Part model, mm, in its own coordinate system. Face numbers are marked on the shaded views. A direction names the side the tool comes from. Round coordinates to 2 decimals unless told otherwise and drop trailing zeros. Loops run counter-clockwise (first coordinate to the right, second up) from the corner with the lowest first, then second, coordinate; pieces in that order, holes last. Notation, with made-up numbers: (88.5, 33.5) - (132.5, 33.5) arc R9 ccw to (132.5, 40.5) - close; hole circle Ø5 at (31.5, 37). An arc over 180 degrees is marked (long way). Put each result on its own line as item: value.
from build123d import *

# Parameters (mm, degrees)
SKETCH1_W                  = 76.2
SKETCH1_H                  = 63.5
BOSS_EXTRUDE1_DEPTH        = 14.2875
SKETCH2_W                  = 50.8
SKETCH2_H                  = 36.1
CUT_EXTRUDE1_DEPTH         = 19.05
M10X1_5_TAPPED_HOLE1_D     = 8.5
M10X1_5_TAPPED_HOLE1_DEPTH = 22.446342369
M10X1_5_TAPPED_HOLE1_TIP   = 2.553657631
SKETCH16_W                 = 3.724215622
SKETCH16_H                 = 1.92405
FILLET2_R                  = 3.175
F_4_40_TAPPED_HOLE2_D      = 2.2606
F_4_40_TAPPED_HOLE2_DEPTH  = 6.920847242
F_4_40_TAPPED_HOLE2_TIP    = 0.679152758
FILLET3_R                  = 4
F_4_40_TAPPED_HOLE3_D      = 2.2606
F_4_40_TAPPED_HOLE3_DEPTH  = 4.320847242
F_4_40_TAPPED_HOLE3_TIP    = 0.679152758
F_8_32_TAPPED_HOLE1_D      = 3.4544
F_8_32_TAPPED_HOLE1_DEPTH  = 9.672193539
F_8_32_TAPPED_HOLE1_TIP    = 1.037806461


with BuildPart() as part:
    # Sketch1 → Boss-Extrude1 (new body, symmetric)
    with BuildSketch(Plane(origin=(0, 0, 0), x_dir=(1, 0, 0), z_dir=(0, 1, 0))):
        Rectangle(SKETCH1_W, SKETCH1_H)
    extrude(amount=BOSS_EXTRUDE1_DEPTH, both=True)

    # Sketch2 → Cut-Extrude1 (cut)
    with BuildSketch(Plane(origin=(0, 14.2875, 0), x_dir=(1, 0, 0), z_dir=(0, 1, 0))):
        Rectangle(SKETCH2_W, SKETCH2_H)
    extrude(amount=-CUT_EXTRUDE1_DEPTH, mode=Mode.SUBTRACT)

    # M10x1.5 Tapped Hole1
    with Locations(Plane(origin=(-21.9, 4.2875, -31.75), x_dir=(-1, 0, 0), z_dir=(0, 0, -1))):
        with Locations((0, 0)):
            Hole(M10X1_5_TAPPED_HOLE1_D / 2, depth=M10X1_5_TAPPED_HOLE1_DEPTH)
            with Locations((0, 0, -(M10X1_5_TAPPED_HOLE1_DEPTH + M10X1_5_TAPPED_HOLE1_TIP / 2))):  # 118° drill point
                Cone(0, M10X1_5_TAPPED_HOLE1_D / 2, M10X1_5_TAPPED_HOLE1_TIP, mode=Mode.SUBTRACT)

    # Cut-Sweep1: sweep along a path in Sketch14
    with BuildLine(Plane(origin=(0, 14.2875, 0), x_dir=(1, 0, 0), z_dir=(0, 1, 0))) as cut_sweep1_path:
        Line((-21.4, 20.05), (21.4, 20.05))
        ThreePointArc((21.4, 20.05), (25.642640687, 18.292640687), (27.4, 14.05))
        Line((27.4, 14.05), (27.4, -14.05))
        ThreePointArc((27.4, -14.05), (25.642640687, -18.292640687), (21.4, -20.05))
        Line((21.4, -20.05), (-21.4, -20.05))
        ThreePointArc((-21.4, -20.05), (-25.642640687, -18.292640687), (-27.4, -14.05))
        Line((-27.4, -14.05), (-27.4, 14.05))
        ThreePointArc((-27.4, 14.05), (-25.642640687, 18.292640687), (-21.4, 20.05))
    # Sketch16 → Cut-Sweep1 (sweep, cut)
    with BuildSketch(Plane.XY):
        with Locations((-29.262107811, 13.325475)):
            Rectangle(SKETCH16_W, SKETCH16_H)
    sweep(path=cut_sweep1_path.line, mode=Mode.SUBTRACT)

    # Fillet2
    fillet2_edges = [part.edges().sort_by_distance(p)[0] for p in [
        (38.1, 0, 31.75),
        (-38.1, 0, 31.75),
        (-38.1, 0, -31.75),
        (38.1, 0, -31.75),
    ]]
    fillet(fillet2_edges, radius=FILLET2_R)

    # #4-40 Tapped Hole2
    with Locations(Plane(origin=(0, 14.2875, 0), x_dir=(1, 0, 0), z_dir=(0, 1, 0))):
        with Locations((34.124215622, 0), (30.228658441, 23.222452534), (-30.397379151, 23.047379151), (30.397379151, -23.047379151), (-30.397379151, -23.047379151), (0, -26.774215622), (-34.124215622, 0), (0.004913792, 26.774215622)):
            Hole(F_4_40_TAPPED_HOLE2_D / 2, depth=F_4_40_TAPPED_HOLE2_DEPTH)
            with Locations((0, 0, -(F_4_40_TAPPED_HOLE2_DEPTH + F_4_40_TAPPED_HOLE2_TIP / 2))):  # 118° drill point
                Cone(0, F_4_40_TAPPED_HOLE2_D / 2, F_4_40_TAPPED_HOLE2_TIP, mode=Mode.SUBTRACT)

    # Fillet3
    fillet3_edges = [part.edges().sort_by_distance(p)[0] for p in [
        (25.4, 4.7625, -18.05),
        (25.4, 4.7625, 18.05),
        (-25.4, 4.7625, 18.05),
        (-25.4, -1.442956345, -18.05),
        (-25.4, 10.492956345, -18.05),
    ]]
    fillet(fillet3_edges, radius=FILLET3_R)

    # #4-40 Tapped Hole3
    with Locations(Plane(origin=(19.4, -4.7625, -12.05), x_dir=(0, 0, 1), z_dir=(0, 1, 0))):
        with Locations((0, 0), (24.1, 0), (24.1, -38.8), (0, -38.8)):
            Hole(F_4_40_TAPPED_HOLE3_D / 2, depth=F_4_40_TAPPED_HOLE3_DEPTH)
            with Locations((0, 0, -(F_4_40_TAPPED_HOLE3_DEPTH + F_4_40_TAPPED_HOLE3_TIP / 2))):  # 118° drill point
                Cone(0, F_4_40_TAPPED_HOLE3_D / 2, F_4_40_TAPPED_HOLE3_TIP, mode=Mode.SUBTRACT)

    # #8-32 Tapped Hole1
    with Locations(Plane.XZ.offset(14.2875)):
        with Locations((32.75, -12.7), (-32.75, 12.7), (-32.75, -12.7), (32.75, 12.7)):
            Hole(F_8_32_TAPPED_HOLE1_D / 2, depth=F_8_32_TAPPED_HOLE1_DEPTH)
            with Locations((0, 0, -(F_8_32_TAPPED_HOLE1_DEPTH + F_8_32_TAPPED_HOLE1_TIP / 2))):  # 118° drill point
                Cone(0, F_8_32_TAPPED_HOLE1_D / 2, F_8_32_TAPPED_HOLE1_TIP, mode=Mode.SUBTRACT)


solid = part.part
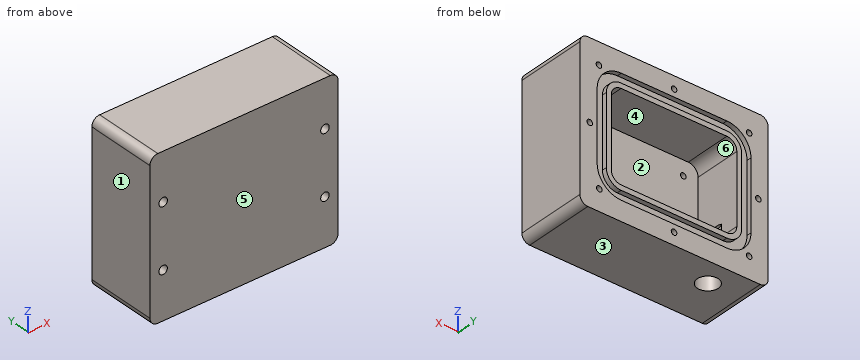
1. Band-saw the part on B-B (x = 8.5). List the corners of the cut face in (y, z), plus the area to 3 significant figures.
A:
outline: (-14.29, -31.75) - (14.29, -31.75) - (14.29, -23.77) - (12.36, -23.77) - (12.36, -20.05) - (14.29, -20.05) - (14.29, -18.05) - (-4.76, -18.05) - (-4.76, 18.05) - (14.29, 18.05) - (14.29, 20.05) - (12.36, 20.05) - (12.36, 23.77) - (14.29, 23.77) - (14.29, 31.75) - (-14.29, 31.75) - close
area: 1,110 mm²
2. Band-saw the part on C-C (z = 15.5). List the corners of the cut face in (x, y).
A:
outline: (-38.1, -14.29) - (38.1, -14.29) - (38.1, 14.29) - (31.02, 14.29) - (31.02, 12.36) - (27.22, 12.36) - (27.22, 14.29) - (25.13, 14.29) - (25.13, -4.76) - (-25.13, -4.76) - (-25.13, 14.29) - (-27.22, 14.29) - (-27.22, 12.36) - (-31.02, 12.36) - (-31.02, 14.29) - (-38.1, 14.29) - close
3. Two-plate mould, pull along X, no slides. Class the marked faces 1, 2, 3 and 4: pulls with the +X half, pulls with the -X half, needs draft (parallel to the pull), parting line crosses it, or undercut.
A:
face 1: pulls with the -X half
face 2: undercut
face 3: needs draft
face 4: undercut
4. Tool access for the marked faces 5 and 6: list every direction of +Z, -Z, +X, -X, +Y, -Y with a clear straight run to the whole face (end or side of a thin tool).
A:
face 5: +Z, -Z, +X, -X, -Y
face 6: +Y
5. Probe line 1 along Z through (x, y) = (-10.5, 13); line 2 along Z through (x, y) = (19.4, -6.7); line 3 along Z through (x, y) = (3, 9.75). List the from-to ranges inside material, lowest first. Write a range as [from, to].
A:
line 1: z = [-31.75, -23.77], [-20.05, -18.05], [18.05, 20.05], [23.77, 31.75]
line 2: z = [-31.75, -13.18], [-10.92, 10.92], [13.18, 31.75]
line 3: z = [-31.75, -18.05], [18.05, 31.75]
6. Band-saw the part on A-A (y = -1). List the corners of the cut face in (x, z) (3 decimals).
A:
outline: (-38.1, -28.575) arc R3.175 ccw to (-34.925, -31.75) - (34.925, -31.75) arc R3.175 ccw to (38.1, -28.575) - (38.1, 28.575) arc R3.175 ccw to (34.925, 31.75) - (-34.925, 31.75) arc R3.175 ccw to (-38.1, 28.575) - close; hole (-25.4, -14.05) arc R4 ccw to (-21.4, -18.05) - (21.4, -18.05) arc R4 ccw to (25.4, -14.05) - (25.4, 14.05) arc R4 ccw to (21.4, 18.05) - (-21.4, 18.05) arc R4 ccw to (-25.4, 14.05) - close
